The listing builds one solid part. Answer for the finished solid, in the listing's coordinates (mm). Face numbers are marked on the shaded views. A direction names the side the tool comes from. Give positions to 0.01 mm unless a question says otherwise; leave off trailing zeros. Order: outer loops, then holes, each group sorted by start corner. A loop starts at its lowest first (then second) coordinate and runs counter-clockwise, first axis right, second up. Notation, with made-up numbers: (45, -13.75) - (84, -13.75) arc R37 ccw to (84, 23.25) - close; hole circle Ø3 at (-18, -28). An arc over 180 degrees is marked (long way). Answer as a JSON object with one key per item and string values. Group by question number.
Q1. For the marked faces 1, 2, 3 and 4, determine the directions among +Z, -Z, +X, -X, +Y, -Y from which every point of the face is accessible in a straight line to the end or side of a thin tool.
Q2. A cutting plane is placed at B-B, the plane z = 7.5. Give the vertices of the cut face in (x, y), and give its area (3 significant figures).
Q3. The mould has two halves that part along X. Classify the marked faces 5, 6, 7 and 8: released by +X, released by -X, zero draft, split by the parting line, or undercut.
Q4. Given pin 1 (1.5 mm diameter, centred on x = 4, y = 11, fed in from +Z); pin 2 (6 mm diameter, centred on y = 10.5, z = 14, fed in from +X); pin 3 (2 mm diameter, centred on x = 37, y = 6.5, fed in from +Z); pin 4 (5 mm diameter, centred on x = 15, y = 6.555, fed in from +Z), each flat-ended and moving along its own axis, determine where each tip first touches the part or whether it passes through.
Q5. A cutting plane is placed at D-D, the plane x = 15. Give the vertices of the cut face in (y, z) (3 decimals).
Q6. A cutting plane is placed at A-A, the plane x = -8. Give the vertices of the cut face in (y, z).
Q7. A cutting plane is placed at C-C, the plane z = 1. Give the vertices of the cut face in (x, y), and give its area (3 significant figures).
Q8. Consider line 1 (X direction, y = 7.25, z = 2); line 2 (X direction, y = 3, z = 1.5); line 3 (X direction, y = 1.25, z = -3). Determine where each line is inside the solid, lowest interval first.
from build123d import *

# Parameters (mm, degrees)
P_IDAT_VYSUNUT_M1_DEPTH  = 13
P_IDAT_VYSUNUT_M2_DEPTH  = 13
SKICA3_W                 = 6
SKICA3_H                 = 12.5
ODEBRAT_VYSUNUT_M1_DEPTH = 44.544517451
SKICA4_W                 = 24
SKICA4_H                 = 16
ODEBRAT_VYSUNUT_M2_DEPTH = 12
SKICA5_R                 = 0.9
ODEBRAT_VYSUNUT_M3_DEPTH = 5
ZAOBLIT1_R               = 6.5
SKICA6_R                 = 3.75
ODEBRAT_VYSUNUT_M4_DEPTH = 5
SKICA7_R                 = 4.75
ODEBRAT_VYSUNUT_M5_DEPTH = 5
SKICA8_W                 = 4
SKICA8_H                 = 11
ODEBRAT_VYSUNUT_M6_DEPTH = 5
SKICA9_R                 = 4
ODEBRAT_VYSUNUT_M7_DEPTH = 10
SKICA10_R                = 6
P_IDAT_VYSUNUT_M3_DEPTH  = 0.5
SKICA11_R                = 4.5
P_IDAT_VYSUNUT_M4_DEPTH  = 3
SKICA12_W                = 4
SKICA12_H                = 2
P_IDAT_VYSUNUT_M5_DEPTH  = 13


with BuildPart() as part:
    # Skica1 → Přidat vysunutím1 (new body)
    with BuildSketch(Plane(origin=(0, 0, 0), x_dir=(1, 0, 0), z_dir=(0, 1, 0))):
        Polygon((0, -11), (0, 11), (-3.25, 14.25), (-38.25, 14.25), (-38.25, 16.25), (-2.421572875, 16.25), (2, 11.828427125), (2, -11.828427125), (-2.421572875, -16.25), (-38.25, -16.25), (-38.25, -14.25), (-3.25, -14.25), align=None)
    extrude(amount=P_IDAT_VYSUNUT_M1_DEPTH)

    # Skica2 → Přidat vysunutím2 (add)
    with BuildSketch(Plane.XZ):
        Polygon((0.078427125, 13.75), (35, 13.75), (35, 1.75), (37.5, 1.75), (37.5, -3.25), (2, -3.25), (2, 11.828427125), align=None)
    extrude(amount=-P_IDAT_VYSUNUT_M2_DEPTH)

    # Skica3 → Odebrat vysunutím1 (cut, through all)
    with BuildSketch(Plane(origin=(0, 13, 0), x_dir=(1, 0, 0), z_dir=(0, 1, 0))):
        with Locations((5, -5.5)):
            Rectangle(SKICA3_W, SKICA3_H)
    extrude(amount=-ODEBRAT_VYSUNUT_M1_DEPTH, mode=Mode.SUBTRACT)

    # Skica4 → Odebrat vysunutím2 (cut)
    with BuildSketch(Plane(origin=(0, 13, 0), x_dir=(1, 0, 0), z_dir=(0, 1, 0))):
        with Locations((21.5, -4.75)):
            Rectangle(SKICA4_W, SKICA4_H)
    extrude(amount=-ODEBRAT_VYSUNUT_M2_DEPTH, mode=Mode.SUBTRACT)

    # Skica5 → Odebrat vysunutím3 (cut)
    with BuildSketch(Plane(origin=(0, 0, -3.25), x_dir=(-1, 0, 0), z_dir=(0, 0, -1))):
        with Locations((-34.993787626, 6.555058734)):
            Circle(SKICA5_R)
        with Locations((-8.006314188, 6.5550616)):
            Circle(SKICA5_R)
    extrude(amount=-ODEBRAT_VYSUNUT_M3_DEPTH, mode=Mode.SUBTRACT)

    # Zaoblit1
    zaoblit1_edges = [part.edges().sort_by_distance(p)[0] for p in [
        (-38.25, 0, -15.25),
        (-38.25, 0, 15.25),
        (-38.25, 13, 15.25),
        (-38.25, 13, -15.25),
    ]]
    fillet(zaoblit1_edges, radius=ZAOBLIT1_R - 0.0001)  # a hair under: the kernel refuses the full size

    # Skica6 → Odebrat vysunutím4 (cut)
    with BuildSketch(Plane(origin=(0, 0, -16.25), x_dir=(-1, 0, 0), z_dir=(0, 0, -1))):
        with Locations((31.75, 6.5)):
            Circle(SKICA6_R)
    extrude(amount=-ODEBRAT_VYSUNUT_M4_DEPTH, mode=Mode.SUBTRACT)

    # Skica7 → Odebrat vysunutím5 (cut)
    with BuildSketch(Plane(origin=(0, 0, 14.25), x_dir=(-1, 0, 0), z_dir=(0, 0, -1))):
        with Locations((31.75, 6.5)):
            Circle(SKICA7_R)
    extrude(amount=-ODEBRAT_VYSUNUT_M5_DEPTH, mode=Mode.SUBTRACT)

    # Skica8 → Odebrat vysunutím6 (cut)
    with BuildSketch(Plane(origin=(35, 0, 0), x_dir=(0, 0, -1), z_dir=(1, 0, 0))):
        with Locations((-10.25, 7.5)):
            Rectangle(SKICA8_W, SKICA8_H)
    extrude(amount=-ODEBRAT_VYSUNUT_M6_DEPTH, mode=Mode.SUBTRACT)

    # Skica9 → Odebrat vysunutím7 (cut)
    with BuildSketch(Plane.XY.offset(13.75)):
        with Locations((15, 6.554999832)):
            Circle(SKICA9_R)
    extrude(amount=-ODEBRAT_VYSUNUT_M7_DEPTH, mode=Mode.SUBTRACT)

    # Skica10 → Přidat vysunutím3 (add)
    with BuildSketch(Plane.XY.offset(13.75)):
        with Locations((27.118831388, 6.554999832)):
            Circle(SKICA10_R)
    extrude(amount=P_IDAT_VYSUNUT_M3_DEPTH)

    # Skica11 → Přidat vysunutím4 (add)
    with BuildSketch(Plane.XY.offset(14.25)):
        with Locations((27.118831388, 6.554999832)):
            Circle(SKICA11_R)
    extrude(amount=P_IDAT_VYSUNUT_M4_DEPTH)

    # Skica12 → Přidat vysunutím5 (add)
    with BuildSketch(Plane(origin=(0, 13, 0), x_dir=(1, 0, 0), z_dir=(0, 1, 0))):
        with Locations((-15, 13.25)):
            Rectangle(SKICA12_W, SKICA12_H)
    extrude(amount=-P_IDAT_VYSUNUT_M5_DEPTH)


solid = part.part
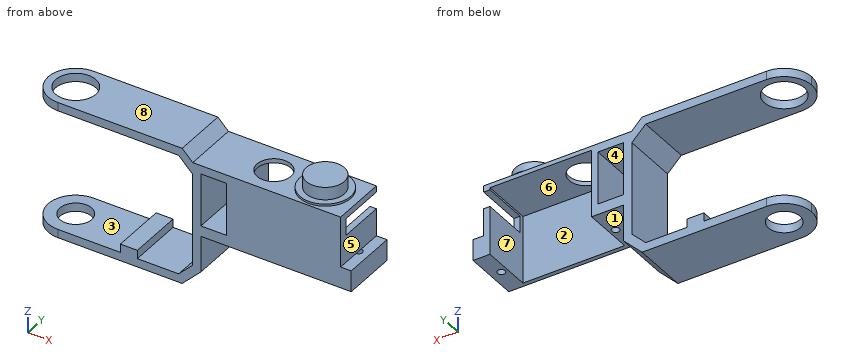
Reply:
{
 "1": {"face 1": "-Z, +X, +Y, -Y", "face 2": "-Z, +Y", "face 3": "-X, +Y, -Y", "face 4": "+Y, -Y"},
 "2": {"outline": "(0, 0) - (2, 0) - (2, 13) - (0, 13) - close; (8, 0) - (35, 0) - (35, 13) - (33.5, 13) - (33.5, 1) - (9.5, 1) - (9.5, 13) - (8, 13) - close", "area": "89.0 mm^2"},
 "3": {"face 5": "released by +X", "face 6": "undercut", "face 7": "undercut", "face 8": "zero draft"},
 "4": {"pin 1": "stops at z = 13.75", "pin 2": "stops at x = 35", "pin 3": "stops at z = 1.75", "pin 4": "passes through"},
 "5": {"outline": "(0, -3.25) - (1, -3.25) - (1, 12.75) - (2.555, 12.75) - (2.555, 13.75) - (0, 13.75) - close; (10.555, 12.75) - (13, 12.75) - (13, 13.75) - (10.555, 13.75) - close"},
 "6": {"outline": "(0, -16.25) - (13, -16.25) - (13, -14.25) - (0, -14.25) - close; (0, 14.25) - (13, 14.25) - (13, 16.25) - (0, 16.25) - close"},
 "7": {"outline": "(0, 0) - (2, 0) - (2, 13) - (0, 13) - close; (8, 0) - (37.5, 0) - (37.5, 13) - (33.5, 13) - (33.5, 1) - (9.5, 1) - (9.5, 13) - (8, 13) - (8, 7.46) arc R0.9 cw (long way) to (8, 5.66) - close; hole circle Ø1.8 at (34.99, 6.56)", "area": "118 mm^2"},
 "8": {"line 1": "x = 0 to 2, 8 to 9.5, 33.5 to 35", "line 2": "x = 0 to 2, 8 to 9.5, 33.5 to 37.5", "line 3": "x = 0 to 9.5, 33.5 to 37.5"}
}
